Build history of the part. All positions in model axes, mm. A direction names the side the tool comes from. Give positions to 0.01 mm unless a question says otherwise; leave off trailing zeros. Write each loop counter-clockwise with the first axis right and the second up, starting at its lowest first coordinate (ties: lowest second). Pieces come first, ordered by that corner, then holes. Notation, with made-up numbers: (43, 44) -> (66, 44) arc R27 ccw to (66, 63) -> close; hole circle Ø6 at (-30.75, 76). An arc over 180 degrees is marked (long way). Put each result on its own line as item: value. Start each with the question number.
Item 1: Tool access for faces 1 (the flat face through (-100, 16, 1)), 2 (the cylindrical face through (11.99, 25.85, 48.48)): list every direction of +Z, -Z, +X, -X, +Y, -Y with a clear straight run to the whole face (end or side of a thin tool).
Item 2: Slice it at D-D, the plane z = -41.5. List the corners of the cut face in (x, y), plus the area to 3 significant figures.
Item 3: Two-plate mould, pull along Z, no slides. Class faces 3 (the cylindrical face through (-98.52, 36.36, 1.34)), 4 (the flat face through (-1, 3, -6)), 5 (the flat face through (9.4, 23.8, 47)), 6 (the flat face through (-71, 2, 30)): pulls with the +Z half, pulls with the -Z half, needs draft (parallel to the pull), parting line crosses it, or undercut.
Item 4: Drill centre lines: line 1 along Y through (x, z) = (-98, 0); line 2 along Y through (x, z) = (65, 7.5); line 3 along X through (y, z) = (9, 11). Where is each one in solid material? Low to high.
Item 5: Flat gauge pins, fed straight in: pin 1 Ø11.5 at (y, z) = (23, 0) entering from +X; pin 2 Ø0.9 at (x, z) = (-0.5, 49) entering from +Y; pin 3 Ø2.5 at (y, z) = (40, 48) entering from +X; pin 4 Ø1 at (x, z) = (-15.5, 2) entering from +Y. Where does each tip first touch, or does it go through?
Item 6: Slice it at C-C, the plane z = 27.5. List the corners of the cut face in (x, y).
Item 7: Slice it at B-B, the plane x = -1. List the corners of the cut face in (y, z), plus the area to 4 significant figures.
Item 8: Slice it at A-A, the plane z = -11.25. List the corners of the cut face in (x, y).
```python
from build123d import *

# Parameters (mm, degrees)
SKETCH1_W                = 200
SKETCH1_H                = 100
BOSS_EXTRUDE1_DEPTH      = 3
BOSS_EXTRUDE2_DEPTH      = 50
CUT_EXTRUDE1_DEPTH       = 50
CUT_EXTRUDE2_DEPTH       = 152.026487743
CUT_EXTRUDE2_DEPTH_BACK  = 152.026487743
BOSS_EXTRUDE4_DEPTH      = 30
SKETCH7_R                = 6.5
CUT_EXTRUDE4_DEPTH       = 220
SKETCH8_W                = 3
SKETCH8_H                = 40
BOSS_EXTRUDE5_DEPTH      = 10
SKETCH9_R                = 2.5
CUT_EXTRUDE5_DEPTH       = 247
CUT_EXTRUDE6_DEPTH       = 29
CUT_EXTRUDE7_DEPTH       = 29
SKETCH12_W               = 90
SKETCH12_H               = 10
CUT_EXTRUDE9_DEPTH       = 3
BOSS_EXTRUDE6_DEPTH      = 90
CUT_EXTRUDE10_DEPTH      = 90
CUT_EXTRUDE11_DEPTH      = 90
CUT_EXTRUDE12_DEPTH      = 217.5
CUT_EXTRUDE14_DEPTH      = 59
CUT_EXTRUDE14_DEPTH_BACK = 122


with BuildPart() as part:
    # Sketch1 → Boss-Extrude1 (new body)
    with BuildSketch(Plane(origin=(0, 0, 0), x_dir=(1, 0, 0), z_dir=(0, 1, 0))):
        Rectangle(SKETCH1_W, SKETCH1_H)
    extrude(amount=BOSS_EXTRUDE1_DEPTH)

    # Sketch2 → Boss-Extrude2 (add)
    with BuildSketch(Plane(origin=(0, 3, 0), x_dir=(1, 0, 0), z_dir=(0, 1, 0))):
        Polygon((0, -50), (-45, -50), (-45, -47), (45, -47), (45, -50), align=None)
    extrude(amount=BOSS_EXTRUDE2_DEPTH)

    # Sketch3 → Cut-Extrude1 (cut)
    with BuildSketch(Plane.XY.offset(50)):
        with BuildLine():
            ThreePointArc((-32.889241728, 44.970705016), (-34.967685824, 31.496355047), (-31.740232125, 18.250163911))
            ThreePointArc((-31.740232125, 18.250163911), (-28.419512967, 17.036564194), (-27.20591325, 20.357283352))
            ThreePointArc((-27.20591325, 20.357283352), (-29.972302134, 31.711161468), (-28.190778624, 43.2606043))
            ThreePointArc((-28.190778624, 43.2606043), (-29.684959817, 46.46488621), (-32.889241728, 44.970705016))
        make_face()
        with BuildLine():
            ThreePointArc((27.20591325, 20.357283352), (28.419512967, 17.036564194), (31.740232125, 18.250163911))
            ThreePointArc((31.740232125, 18.250163911), (34.967685824, 31.496355047), (32.889241728, 44.970705016))
            ThreePointArc((32.889241728, 44.970705016), (29.684959817, 46.46488621), (28.190778624, 43.2606043))
            ThreePointArc((28.190778624, 43.2606043), (29.972302134, 31.711161468), (27.20591325, 20.357283352))
        make_face()
    extrude(amount=-CUT_EXTRUDE1_DEPTH, mode=Mode.SUBTRACT)

    # Sketch4 → Cut-Extrude2 (cut, two sides: drawn at the far end of the back side and taken through both)
    with BuildSketch(Plane.XY.offset(50).offset(-CUT_EXTRUDE2_DEPTH_BACK)):
        with BuildLine():
            Line((15, 33), (15, 53))
            Line((15, 53), (-15, 53))
            Line((-15, 53), (-15, 33))
            ThreePointArc((-15, 33), (-12.071067812, 25.928932188), (-5, 23))
            Line((-5, 23), (5, 23))
            ThreePointArc((5, 23), (12.071067812, 25.928932188), (15, 33))
        make_face()
    extrude(amount=CUT_EXTRUDE2_DEPTH + CUT_EXTRUDE2_DEPTH_BACK, mode=Mode.SUBTRACT)

    # Sketch5 → Boss-Extrude4 (add)
    with BuildSketch(Plane(origin=(0, 3, 0), x_dir=(1, 0, 0), z_dir=(0, 1, 0))):
        Polygon((-100, 0), (-100, 20), (-97, 20), (-97, -20), (-100, -20), align=None)
        Polygon((100, 0), (100, 20), (97, 20), (97, -20), (100, -20), align=None)
    extrude(amount=BOSS_EXTRUDE4_DEPTH)

    # Sketch7 → Cut-Extrude4 (cut)
    with BuildSketch(Plane.ZY.offset(100)):
        with Locations((0, 23)):
            Circle(SKETCH7_R)
    extrude(amount=-CUT_EXTRUDE4_DEPTH, mode=Mode.SUBTRACT)

    # Sketch8 → Boss-Extrude5 (add)
    with BuildSketch(Plane(origin=(0, 33, 0), x_dir=(1, 0, 0), z_dir=(0, 1, 0))):
        with Locations((-98.5, 0)):
            Rectangle(SKETCH8_W, SKETCH8_H)
        with Locations((98.5, 0)):
            Rectangle(SKETCH8_W, SKETCH8_H)
    extrude(amount=BOSS_EXTRUDE5_DEPTH)

    # Sketch9 → Cut-Extrude5 (cut)
    with BuildSketch(Plane.ZY.offset(100)):
        with Locations((0, 34.25)):
            Circle(SKETCH9_R)
        with Locations((-11.25, 23)):
            Circle(SKETCH9_R)
        with Locations((0, 11.75)):
            Circle(SKETCH9_R)
        with Locations((11.25, 23)):
            Circle(SKETCH9_R)
    extrude(amount=-CUT_EXTRUDE5_DEPTH, mode=Mode.SUBTRACT)

    # Sketch10 → Cut-Extrude6 (cut)
    with BuildSketch(Plane(origin=(0, 3, 0), x_dir=(1, 0, 0), z_dir=(0, 1, 0))):
        Polygon((-45, -50), (-100, -20), (-100, -50), align=None)
    extrude(amount=-CUT_EXTRUDE6_DEPTH, mode=Mode.SUBTRACT)

    # Sketch11 → Cut-Extrude7 (cut)
    with BuildSketch(Plane(origin=(0, 3, 0), x_dir=(1, 0, 0), z_dir=(0, 1, 0))):
        Polygon((45, -50), (100, -20), (100, -50), align=None)
    extrude(amount=-CUT_EXTRUDE7_DEPTH, mode=Mode.SUBTRACT)

    # Sketch12 → Cut-Extrude9 (cut)
    with BuildSketch(Plane.XY.offset(50)):
        with Locations((0, 8)):
            Rectangle(SKETCH12_W, SKETCH12_H)
    extrude(amount=-CUT_EXTRUDE9_DEPTH, mode=Mode.SUBTRACT)


with BuildPart() as cut_extrude9_piece_1:
    # of the separate pieces the step leaves, piece 1, a body of its own (cut_extrude9_pieces)
    add(part.part.solids().sort_by_distance((100, 0, -50))[0])



with BuildPart() as cut_extrude9_piece_2:
    # of the separate pieces the step leaves, piece 2, a body of its own (cut_extrude9_pieces)
    add(part.part.solids().sort_by_distance((-45, 13, 47))[0])


with BuildPart() as cut_extrude9_piece_1_1:
    add(cut_extrude9_piece_1.part)

    add(cut_extrude9_piece_2.part)  # Boss-Extrude6 merges Cut-Extrude9 piece 2
    # Sketch13 → Boss-Extrude6 (add)
    with BuildSketch(Plane.ZY.offset(45)):
        Polygon((47, 13), (37, 3), (47, 3), (50, 3), (50, 13), align=None)
    extrude(amount=-BOSS_EXTRUDE6_DEPTH)

    # Sketch14 → Cut-Extrude10 (cut)
    with BuildSketch(Plane.ZY.offset(45)):
        Polygon((50, 13), (40, 3), (50, 3), align=None)
    extrude(amount=-CUT_EXTRUDE10_DEPTH, mode=Mode.SUBTRACT)

    # Sketch15 → Cut-Extrude11 (cut)
    with BuildSketch(Plane(origin=(0, 3, 0), x_dir=(1, 0, 0), z_dir=(0, 1, 0))):
        Polygon((-100, -20), (-97, -20), (-45, -40), (45, -40), (97, -20), (100, -20), (45, -50), (-45, -50), align=None)
    extrude(amount=-CUT_EXTRUDE11_DEPTH, mode=Mode.SUBTRACT)

    # Sketch16 → Cut-Extrude12 (cut)
    with BuildSketch(Plane.ZY.offset(100)):
        with BuildLine():
            Line((-3.2e-08, 43), (-20, 43))
            Line((-20, 43), (-20, 23))
            ThreePointArc((-20, 23), (-14.142135635, 37.142135612), (-3.2e-08, 43))
        make_face()
        with BuildLine():
            Line((20, 43), (-3.2e-08, 43))
            ThreePointArc((-3.2e-08, 43), (14.142135612, 37.142135635), (20, 23))
            Line((20, 23), (20, 43))
        make_face()
    extrude(amount=-CUT_EXTRUDE12_DEPTH, mode=Mode.SUBTRACT)

    # Sketch17 → Cut-Extrude14 (cut, two sides: drawn at the far end of the back side and taken through both)
    with BuildSketch(Plane.ZY.offset(45).offset(-CUT_EXTRUDE14_DEPTH_BACK)):
        Polygon((40, 3), (40, 0), (37, 0), align=None)
    extrude(amount=CUT_EXTRUDE14_DEPTH + CUT_EXTRUDE14_DEPTH_BACK, mode=Mode.SUBTRACT)


solid = cut_extrude9_piece_1_1.part
```
Values follow:
1. face 1: +Z, -Z, -X, +Y, -Y
1. face 2: +Z, -Z, +Y
2. outline: (-100, 0) -> (100, 0) -> (100, 3) -> (-100, 3) -> close
2. area: 600 mm2
3. face 3: undercut
3. face 4: needs draft
3. face 5: pulls with the -Z half
3. face 6: pulls with the +Z half
4. line 1: 0 to 9.25, 14.25 to 16.5, 29.5 to 31.75, 36.75 to 43
4. line 2: 0 to 3
4. line 3: -100 to -97, 97 to 100
5. pin 1: through
5. pin 2: y = 23
5. pin 3: x = 45
5. pin 4: y = 3
6. outline: (-77.5, 0) -> (77.5, 0) -> (77.5, 3) -> (-77.5, 3) -> close
7. outline: (0, -50) -> (3, -50) -> (3, 37) -> (13, 47) -> (23, 47) -> (23, 50) -> (13, 50) -> (0, 37) -> close
7. area: 325.5 mm2
8. outline: (-100, 0) -> (100, 0) -> (100, 20.5) -> (97, 20.5) -> (97, 3) -> (-97, 3) -> (-97, 20.5) -> (-100, 20.5) -> close; (-100, 25.5) -> (-97, 25.5) -> (-97, 39.54) -> (-100, 39.54) -> close; (97, 25.5) -> (100, 25.5) -> (100, 39.54) -> (97, 39.54) -> close
